For this review, take the finished solid that the model builds, in its own axes (mm). Face numbers are marked on the shaded views. A direction names the side the tool comes from. Coordinates: 2 decimals unless noted, no trailing zeros. Loops run counter-clockwise (first coordinate to the right, second up) from the corner with the lowest first, then second, coordinate; pieces in that order, holes last. Notation, with made-up numbers: M 58.25,61 L 81.25,61 A20 cw 81.25,89 Z; hole C 89.25,2.25 d10. An arc over 180 degrees is marked long. Put each result on its own line as item: value.
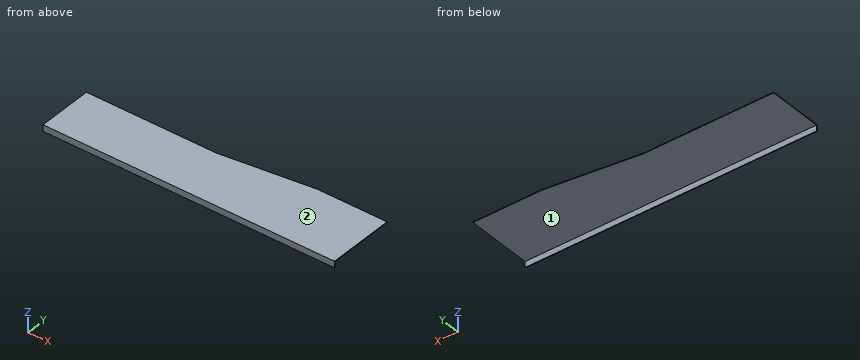
```python
from build123d import *

# Parameters (mm, degrees)
BOSS_EXTRUDE1_DEPTH = 1.27
SKETCH2_W           = 630
SKETCH2_H           = 1.27
BOSS_EXTRUDE2_DEPTH = 13.77


with BuildPart() as part:
    # Sketch1 → Boss-Extrude1 (new body)
    with BuildSketch(Plane.XY):
        Polygon((0, 0), (0, 118.73), (280, 118.73), (480, 143.73), (630, 143.73), (630, 0), align=None)
    extrude(amount=BOSS_EXTRUDE1_DEPTH)

    # Sketch2 → Boss-Extrude2 (add)
    with BuildSketch(Plane.XY.offset(1.27)):
        with Locations((315, 0.635)):
            Rectangle(SKETCH2_W, SKETCH2_H)
    extrude(amount=-BOSS_EXTRUDE2_DEPTH)


solid = part.part
```
(1) For pin 1 (6 mm diameter, centred on y = 64.5, z = -1, fed in from +X); pin 2 (1 mm diameter, centred on x = 73, z = 0.5, fed in from +Y); pin 3 (2 mm diameter, centred on x = 70, y = 31.5, fed in from -Z), all flat-tipped, find the tip position at first contact; note any pin that passes through.
Determined:
pin 1: stops at x = 630
pin 2: stops at y = 118.73
pin 3: stops at z = 0
(2) Tool access review of the marked faces 1 and 2: name each direction out of +Z, -Z, +X, -X, +Y, -Y from which nothing blocks a thin tool from reaching the whole face with its end or side.
Determined:
face 1: -Z, +X, -X, +Y
face 2: +Z, +X, -X, +Y, -Y
(3) Wall thickness on line 1 along Y through (x, z) = (601, -2.5); line 2 along Y through (x, z) = (211, 0.5): over which ranges is each line inside the solid? List them lowest first. Write a range as [from, to].
Determined:
line 1: y = [0, 1.27]
line 2: y = [0, 118.73]
(4) Add section D-D (x = 452). Write out the cut boundary in (y, z), plus the area to 3 significant figures.
Determined:
outline: M 0,-12.5 L 1.27,-12.5 L 1.27,0 L 140.23,0 L 140.23,1.27 L 0,1.27 Z
area: 194 mm^2
(5) Add section B-B (y = 13.5). Write out the cut boundary in (x, z), plus the area to 3 significant figures.
Determined:
outline: M 0,0 L 630,0 L 630,1.27 L 0,1.27 Z
area: 800 mm^2
(6) Add section A-A (x = 216.5). Write out the cut boundary in (y, z), plus the area to 3 significant figures.
Determined:
outline: M 0,-12.5 L 1.27,-12.5 L 1.27,0 L 118.73,0 L 118.73,1.27 L 0,1.27 Z
area: 167 mm^2
